Input: dimensioned drawing with shaded views. Units: mm. Origin: part minimum x, y, z. A direction names the side the tool comes from. Give positions to 0.01 mm unless a question says otherwise; leave off trailing zeros. Order: outer loops, then holes, each group sorted by start corner. A loop starts at its lowest first (then second) coordinate and runs counter-clockwise, first axis right, second up. Notation, with made-up numbers: (-26, 72.25) - (26, 72.25) arc R21 cw to (26, 91.25) - close; hole circle Ø6 at (-15, 77.5). An arc over 180 degrees is marked (long way). Use a Markdown table: item, result.
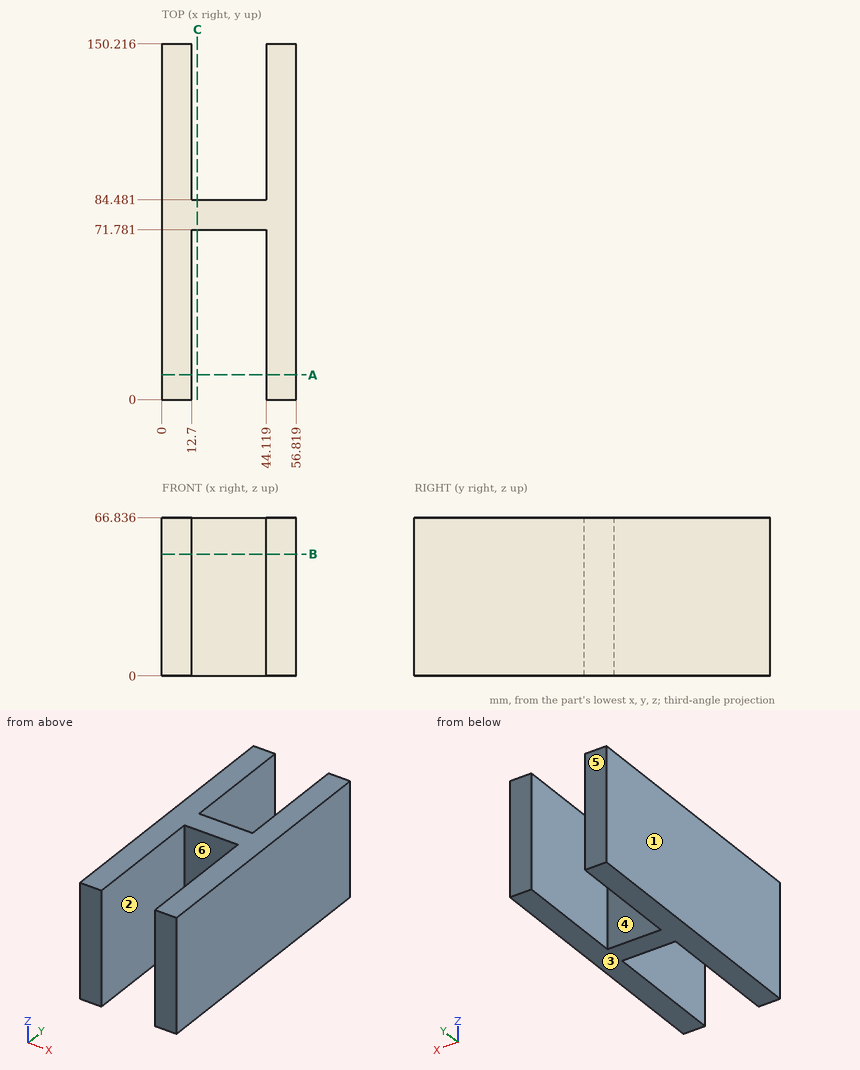
1. Section query B-B (z = 51.5). Return loops of the section in (x, y) (1 decimal).
Response:
| item | result |
|---|---|
| outline | (0, 0) - (12.7, 0) - (12.7, 71.8) - (44.1, 71.8) - (44.1, 0) - (56.8, 0) - (56.8, 150.2) - (44.1, 150.2) - (44.1, 84.5) - (12.7, 84.5) - (12.7, 150.2) - (0, 150.2) - close |
2. Section query C-C (x = 15). Return loops of the section in (y, z), then the cut area to 3 significant figures.
Response:
| item | result |
|---|---|
| outline | (71.78, 0) - (84.48, 0) - (84.48, 66.84) - (71.78, 66.84) - close |
| area | 849 mm^2 |
3. Material intervals for line 1 along X through (y, z) = (64.5, 64); line 2 along Y through (x, z) = (44, 61), sorted ascending.
Response:
| item | result |
|---|---|
| line 1 | x = 0 to 12.7, 44.12 to 56.82 |
| line 2 | y = 71.78 to 84.48 |
4. Set-up query: the marked faces 4, 5 and 6. Return all of +Z, -Z, +X, -X, +Y, -Y with unobstructed straight access to the full face (end or side cutting, diameter ignored); none if empty.
Response:
| item | result |
|---|---|
| face 4 | +Z, -Z, +Y |
| face 5 | +Z, -Z, +X, -X, +Y |
| face 6 | +Z, -Z, -Y |
5. Mould query, pull axis X, two halves, no side actions, for the marked faces 1, 2 and 3. Classes: pulls with the +X half, pulls with the -X half, needs draft (parallel to the pull), parting line crosses it, or undercut.
Response:
| item | result |
|---|---|
| face 1 | pulls with the -X half |
| face 2 | undercut |
| face 3 | needs draft |
6. Section query A-A (y = 10.5). Return loops of the section in (x, z).
Response:
| item | result |
|---|---|
| outline | (0, 0) - (12.7, 0) - (12.7, 66.84) - (0, 66.84) - close; (44.12, 0) - (56.82, 0) - (56.82, 66.84) - (44.12, 66.84) - close |
7. Pin query (flat end, axial travel): pin 1 (2 mm diameter, centred on x = 39.5, z = 35, fed in from +Y). Return the tip coordinate at first contact, or that it passes through.
Response:
| item | result |
|---|---|
| pin 1 | stops at y = 84.48 |
